```python
from build123d import *

# Parameters (mm, degrees)
SKETCH1_W           = 250
SKETCH1_H           = 220
BOSS_EXTRUDE1_DEPTH = 3.175
SKETCH2_R           = 3.2
CUT_EXTRUDE1_DEPTH  = 4.175
FILLET1_R           = 8
CUT_EXTRUDE3_DEPTH  = 4.175
FILLET3_R           = 8
SKETCH5_R           = 8.25
CUT_EXTRUDE4_DEPTH  = 4.175
FILLET4_R           = 10
FILLET5_R           = 8
BOSS_EXTRUDE2_DEPTH = 3.175
FILLET6_R           = 10
SKETCH7_R           = 3.2
CUT_EXTRUDE5_DEPTH  = 4.175


with BuildPart() as part:
    # Sketch1 → Boss-Extrude1 (new body)
    with BuildSketch(Plane(origin=(0, 0, 0), x_dir=(1, 0, 0), z_dir=(0, 1, 0))):
        Rectangle(SKETCH1_W, SKETCH1_H)
    extrude(amount=BOSS_EXTRUDE1_DEPTH)

    # Sketch2 → Cut-Extrude1 (cut, through all)
    with BuildSketch(Plane(origin=(0, 3.175, 0), x_dir=(-1, 0, 0), z_dir=(0, 1, 0))):
        with Locations((117, -102)):
            Circle(SKETCH2_R)
        with Locations((-117, -102)):
            Circle(SKETCH2_R)
        with Locations((-117, 102)):
            Circle(SKETCH2_R)
        with Locations((117, 102)):
            Circle(SKETCH2_R)
        with Locations((117, -77)):
            Circle(SKETCH2_R)
        with Locations((117, 77)):
            Circle(SKETCH2_R)
        with Locations((-117, 77)):
            Circle(SKETCH2_R)
        with Locations((-117, -77)):
            Circle(SKETCH2_R)
        with Locations((117, 37)):
            Circle(SKETCH2_R)
        with Locations((117, -37)):
            Circle(SKETCH2_R)
        with Locations((-117, -37)):
            Circle(SKETCH2_R)
        with Locations((-117, 37)):
            Circle(SKETCH2_R)
    extrude(amount=-CUT_EXTRUDE1_DEPTH, mode=Mode.SUBTRACT)

    # Fillet1
    fillet1_edges = [part.edges().sort_by_distance(p)[0] for p in [
        (-125, 1.5875, -110),
        (125, 1.5875, -110),
        (125, 1.5875, 110),
        (-125, 1.5875, 110),
    ]]
    fillet(fillet1_edges, radius=FILLET1_R)

    # Sketch4 → Cut-Extrude3 (cut, through all)
    with BuildSketch(Plane(origin=(0, 3.175, 0), x_dir=(1, 0, 0), z_dir=(0, 1, 0))):
        with BuildLine():
            Line((75, 110), (50, 110))
            ThreePointArc((50, 110), (62.5, 97.5), (75, 110))
        make_face()
    extrude(amount=-CUT_EXTRUDE3_DEPTH, mode=Mode.SUBTRACT)

    # Fillet3
    fillet3_edges = [part.edges().sort_by_distance(p)[0] for p in [
        (75, 1.5875, -110),
        (50, 1.5875, -110),
    ]]
    fillet(fillet3_edges, radius=FILLET3_R)

    # Sketch5 → Cut-Extrude4 (cut, through all)
    with BuildSketch(Plane(origin=(0, 3.175, 0), x_dir=(1, 0, 0), z_dir=(0, 1, 0))):
        with Locations((-125, 57)):
            Circle(SKETCH5_R)
        with Locations((-125, -57)):
            Circle(SKETCH5_R)
        with BuildLine():
            Line((108.641149162, 70.240746381), (117.711258049, 53.135192013))
            ThreePointArc((117.711258049, 53.135192013), (132.069199597, 52.746893247), (125, 65.25))
            Line((125, 65.25), (125, 77.296464556))
            ThreePointArc((125, 77.296464556), (120.427492424, 70.453223368), (112.355339059, 72.058874503))
            Line((112.355339059, 72.058874503), (111.82233047, 72.591883092))
            ThreePointArc((111.82233047, 72.591883092), (109.219390768, 72.786063189), (108.641149162, 70.240746381))
        make_face()
        with BuildLine():
            Line((112.355339059, -72.058874503), (111.82233047, -72.591883092))
            ThreePointArc((111.82233047, -72.591883092), (109.219390768, -72.786063189), (108.641149162, -70.240746381))
            Line((108.641149162, -70.240746381), (117.711258049, -53.135192013))
            ThreePointArc((117.711258049, -53.135192013), (132.069199597, -52.746893247), (125, -65.25))
            Line((125, -65.25), (125, -77.296464556))
            ThreePointArc((125, -77.296464556), (120.427492424, -70.453223368), (112.355339059, -72.058874503))
        make_face()
    extrude(amount=-CUT_EXTRUDE4_DEPTH, mode=Mode.SUBTRACT)

    # Fillet4
    fillet4_edges = [part.edges().sort_by_distance(p)[0] for p in [
        (-125, 1.5875, -65.25),
        (-125, 1.5875, -48.75),
        (-125, 1.5875, 48.75),
        (-125, 1.5875, 65.25),
    ]]
    fillet(fillet4_edges, radius=FILLET4_R)

    # Fillet5
    fillet5_edges = [part.edges().sort_by_distance(p)[0] for p in [
        (125, 1.5875, -48.75),
        (125, 1.5875, 48.75),
    ]]
    fillet(fillet5_edges, radius=FILLET5_R)

    # Sketch6 → Boss-Extrude2 (add)
    with BuildSketch(Plane(origin=(0, 3.175, 0), x_dir=(1, 0, 0), z_dir=(0, 1, 0))):
        with BuildLine():
            Line((125, 65.189169677), (125, 77.296464556))
            Line((125, 77.296464556), (116.645162041, 73.27854658))
            Line((116.645162041, 73.27854658), (108.408116908, 79.390702383))
            Line((108.408116908, 79.390702383), (108.408116908, 56.119015219))
            Line((108.408116908, 56.119015219), (125, 42.85565484))
            Line((125, 42.85565484), (125, 48.810830323))
            ThreePointArc((125, 48.810830323), (117.75, 57), (125, 65.189169677))
        make_face()
        with BuildLine():
            Line((125, -42.85565484), (125, -48.810830323))
            ThreePointArc((125, -48.810830323), (117.75, -57), (125, -65.189169677))
            Line((125, -65.189169677), (125, -77.296464556))
            Line((125, -77.296464556), (116.645162041, -73.27854658))
            Line((116.645162041, -73.27854658), (108.408116908, -79.390702383))
            Line((108.408116908, -79.390702383), (108.408116908, -56.119015219))
            Line((108.408116908, -56.119015219), (125, -42.85565484))
        make_face()
    extrude(amount=-BOSS_EXTRUDE2_DEPTH)

    # Fillet6
    fillet6_edges = [part.edges().sort_by_distance(p)[0] for p in [
        (125, 1.5875, -65.189169677),
        (125, 1.5875, -48.810830323),
        (125, 1.5875, 48.810830323),
        (125, 1.5875, 65.189169677),
    ]]
    fillet(fillet6_edges, radius=FILLET6_R)

    # Sketch7 → Cut-Extrude5 (cut, through all)
    with BuildSketch(Plane(origin=(0, 3.175, 0), x_dir=(1, 0, 0), z_dir=(0, 1, 0))):
        with Locations((117.002495653, 0)):
            Circle(SKETCH7_R)
        with Locations((-117.002495653, 0)):
            Circle(SKETCH7_R)
    extrude(amount=-CUT_EXTRUDE5_DEPTH, mode=Mode.SUBTRACT)


solid = part.part
```
Input: part model. Units: mm. Frame: model coordinates. Round coordinates to 2 decimals unless told otherwise and drop trailing zeros. Loops run counter-clockwise (first coordinate to the right, second up) from the corner with the lowest first, then second, coordinate; pieces in that order, holes last. Notation, with made-up numbers: (-32.75, -27) - (22.25, -27) arc R25 ccw to (22.25, 9) - close; hole circle Ø6 at (82.5, -22). An arc over 180 degrees is marked (long way). One line per item, written item: value. Start each with the question number.
(1) Ray query, line 1 (X direction, y = 1.75, z = 0); line 2 (X direction, y = 2.25, z = -72); line 3 (Z direction, x = 63, y = 1.2). Return the intervals inside material, ascending. Write a range as [from, to].
(2) Contact query for a flat-ended pin moving along its axis: P1, Ø6, axis at x = -117, z = 102, coming from the +Y side. Output: stop coordinate, or through.
(3) Section A-A, the plane z = 77. Return loops of the section in (x, y) (3 decimals).
(4) Draft query along Z for faces 1 (the cylindrical face through (-120.052, 1.61, -101.039)), 2 (the flat face through (-2, 0, -2)), 3 (the cylindrical face through (122.594, 1.61, -107.719)). Return one class per face: +Z half, -Z half, draft (parallel to the pull), parting line (faces both ways), or undercut.
(5) Section C-C, the plane z = -59.5. Return loops of the section in (x, y) (3 decimals), plus the area to 3 significant figures.
(6) Section B-B, the plane y = 2.55. Count the separate pieces of the cut face and the enclosed holes in it, plus the area to 3 significant figures.
Results below:
1. line 1: [-125, -120.2], [-113.8, 113.8], [120.2, 125]
1. line 2: [-125, 125]
1. line 3: [-97.51, 110]
2. P1: through
3. outline: (-125, 0) - (-120.2, 0) - (-120.2, 3.175) - (-125, 3.175) - close; (-113.8, 0) - (113.8, 0) - (113.8, 3.175) - (-113.8, 3.175) - close; (120.2, 0) - (125, 0) - (125, 3.175) - (120.2, 3.175) - close
4. face 1: undercut
4. face 2: draft
4. face 3: -Z half
5. outline: (-117.138, 0) - (118.138, 0) - (118.138, 3.175) - (-117.138, 3.175) - close
5. area: 747 mm^2
6. separate pieces: 1
6. enclosed holes: 14
6. area: 53,800 mm^2
